Autodesk Inventor part; units mm, degrees
ref_plane "YZ Plane" through (0, 0, 0) normal (1, 0, 0) x (0, 1, 0)
ref_plane "XZ Plane" through (0, 0, 0) normal (0, 1, 0) x (-1, 0, 0)
ref_plane "XY Plane" through (0, 0, 0) normal (0, 0, 1) x (1, 0, 0)
sketch "Эскиз1" plane through (0, 0, 0) normal (0, 0, 1) x (1, 0, 0)
  line L0 (-136.1512, -7) -> (-131.1512, -2)
  line L1 (-131.1512, -2) -> (-99.224, -2)
  line L2 (-19, -2) -> (-19, -22)
  line L3 (-19, -22) -> (-24, -27)
  line L4 (-24, -27) -> (-30.8711, -27)
  line L5 (-136.1512, -27) -> (-136.1512, -7)
  line L6 (-141.1512, -58) -> (-75.0711, -58)
  line L7 (-75.0711, -58) -> (-49.0711, -32)
  line L8 (-49.0711, -32) -> (-21.9289, -32)
  line L9 (-21.9289, -32) -> (-14, -24.0711)
  line L10 (-14, -24.0711) -> (-14, 3)
  line L11 (-133.2223, 3) -> (-14, 3)
  line L12 (-133.2223, 3) -> (-141.1512, -4.9289)
  line L13 (-141.1512, -58) -> (-141.1512, -4.9289)
  line L14 (-44.9289, -42) -> (-24.8579, -42)
  line L15 (-24.8579, -42) -> (-45.8579, -63)
  line L16 (-45.8579, -63) -> (-65.9289, -63)
  line L17 (-65.9289, -63) -> (-44.9289, -42)
  line L18 (-4, 3) -> (-9, 3)
  line L19 (-9, 3) -> (-9, -26.1421)
  line L20 (-9, -26.1421) -> (-19.8579, -37)
  line L21 (-19.8579, -37) -> (-47, -37)
  line L22 (-47, -37) -> (-73, -63)
  line L23 (-73, -63) -> (-141.1512, -63)
  line L24 (-141.1512, -67.9) -> (-141.1512, -63)
  line L25 (-47.0828, -36.8) -> (-19.9407, -36.8)
  line L26 (-19.9407, -36.8) -> (-9.2, -26.0593)
  line L27 (-9.2, -26.0593) -> (-9.2, 3.2)
  line L28 (-9.2, 3.2) -> (3.2, 3.2)
  line L29 (3.2, 3.2) -> (3.2, -31.1955)
  line L30 (3.2, -31.1955) -> (-40.7045, -75.1)
  line L31 (-40.7045, -75.1) -> (-141.3512, -75.1)
  line L32 (-141.3512, -75.1) -> (-141.3512, -62.8)
  line L33 (-141.3512, -62.8) -> (-73.0828, -62.8)
  line L34 (-73.0828, -62.8) -> (-47.0828, -36.8)
  line L35 (-21.8461, -32.2) -> (-48.9882, -32.2)
  line L36 (-48.9882, -32.2) -> (-74.9882, -58.2)
  line L37 (-74.9882, -58.2) -> (-141.3512, -58.2)
  line L38 (-141.3512, -58.2) -> (-141.3512, -4.8461)
  line L39 (-141.3512, -4.8461) -> (-133.3051, 3.2)
  line L40 (-133.3051, 3.2) -> (-13.8, 3.2)
  line L41 (-13.8, 3.2) -> (-13.8, -24.1539)
  line L42 (-13.8, -24.1539) -> (-21.8461, -32.2)
  line L43 (-9, 3) -> (-14, 3)
  line L44 (-141.1512, -63) -> (-141.1512, -58)
  line L45 (-99.224, -2) -> (-93.5671, -2)
  line L46 (-93.5671, -2) -> (-86.696, -2)
  line L47 (-86.696, -2) -> (-81.0391, -2)
  line L48 (-81.0391, -2) -> (-74.168, -2)
  line L49 (-74.168, -2) -> (-68.5111, -2)
  line L50 (-68.5111, -2) -> (-61.64, -2)
  line L51 (-61.64, -2) -> (-55.9831, -2)
  line L52 (-55.9831, -2) -> (-49.112, -2)
  line L53 (-49.112, -2) -> (-43.4551, -2)
  line L54 (-43.4551, -2) -> (-36.584, -2)
  line L55 (-36.584, -2) -> (-30.9271, -2)
  line L56 (-30.9271, -2) -> (-19, -2)
  line L57 (-30.8711, -27) -> (-36.528, -27)
  line L58 (-36.528, -27) -> (-43.3991, -27)
  line L59 (-43.3991, -27) -> (-49.056, -27)
  line L60 (-49.056, -27) -> (-55.9271, -27)
  line L61 (-55.9271, -27) -> (-61.584, -27)
  line L62 (-61.584, -27) -> (-68.4551, -27)
  line L63 (-68.4551, -27) -> (-74.112, -27)
  line L64 (-74.112, -27) -> (-80.9831, -27)
  line L65 (-80.9831, -27) -> (-86.64, -27)
  line L66 (-86.64, -27) -> (-93.5111, -27)
  line L67 (-93.5111, -27) -> (-99.168, -27)
  line L68 (-99.168, -27) -> (-106.0391, -27)
  line L69 (-106.0391, -27) -> (-111.696, -27)
  line L70 (-111.696, -27) -> (-136.1512, -27)
  line L71 (-43.6868, -67.9) -> (-141.1512, -67.9)
  line L72 (-4, -28.2132) -> (-43.6868, -67.9)
  line L73 (-4, 3) -> (-4, -28.2132)
  point P0 (-9.2, 3)
  point P1 (-13.8, 3)
  point P2 (-141.1512, -58.2)
  point P3 (-141.1512, -62.8)
  dimension "d15" = 0.2
  dimension "d16" = 0.2
extrude "Выдавливание1" add sketch "Эскиз1" against normal blind 1.5 contours L37 L36 L35 L42 L41 L43 L27 L26 L25 L34 L33 L44
sketch "Эскиз2" plane through (0, 0, 0) normal (0, 0, 1) x (1, 0, 0)
  line L0 (-9.2, -26.0593) -> (-9.2, 3)
  line L1 (-9.2, 3) -> (-13.8, 3)
  line L2 (-13.8, 3) -> (-13.8, -24.1539)
  line L3 (-13.8, -24.1539) -> (-21.8461, -32.2)
  line L4 (-21.8461, -32.2) -> (-48.9882, -32.2)
  line L5 (-48.9882, -32.2) -> (-74.9882, -58.2)
  line L6 (-74.9882, -58.2) -> (-141.1512, -58.2)
  line L7 (-141.1512, -58.2) -> (-141.1512, -62.8)
  line L8 (-141.1512, -62.8) -> (-73.0828, -62.8)
  line L9 (-73.0828, -62.8) -> (-47.0828, -36.8)
  line L10 (-47.0828, -36.8) -> (-19.9407, -36.8)
  line L11 (-19.9407, -36.8) -> (-9.2, -26.0593)
  line L12 (-7.2, -26.8877) -> (-7.2, 5)
  line L13 (-7.2, 5) -> (-15.8, 5)
  line L14 (-15.8, 5) -> (-15.8, -23.3255)
  line L15 (-15.8, -23.3255) -> (-22.6745, -30.2)
  line L16 (-22.6745, -30.2) -> (-49.8167, -30.2)
  line L17 (-49.8167, -30.2) -> (-75.8167, -56.2)
  line L18 (-75.8167, -56.2) -> (-143.1512, -56.2)
  line L19 (-143.1512, -56.2) -> (-143.1512, -64.8)
  line L20 (-143.1512, -64.8) -> (-72.2544, -64.8)
  line L21 (-72.2544, -64.8) -> (-46.2544, -38.8)
  line L22 (-46.2544, -38.8) -> (-19.1123, -38.8)
  line L23 (-19.1123, -38.8) -> (-7.2, -26.8877)
  line L24 (-138.1512, -66.9) -> (-138.1512, -63)
  line L25 (-138.1512, -64.8) -> (-137.8512, -64.8)
  line L26 (-137.8512, -64.8) -> (-137.8512, -56.2)
  line L27 (-5.3, 0) -> (-14, 0)
  line L28 (-7.2, 0) -> (-7.2, -0.3)
  line L29 (-7.2, -0.3) -> (-15.8, -0.3)
  dimension "d17" = 2
  dimension "d18" = 0.3
  dimension "d19" = 0.3
extrude "Выдавливание2" add sketch "Эскиз2" along normal blind 1 contours L11 L10 L9 L8 L26 L6 L5 L4 L3 L2 L29 L0 | L0 L29 L12 L23 L22 L21 L20 L26 L8 L9 L10 L11 | L2 L3 L4 L5 L6 L26 L18 L17 L16 L15 L14 L29
mirror "Зеркальное отражение1" about plane through (-72.5256, -32.55, 1) normal (0, 0, 1) of "Выдавливание2", "Выдавливание1"
sketch "Эскиз3" plane through (0, 0, -1.5) normal (0, 0, -1) x (-1, 0, 0)
  line L0 (163, 30) -> (-28, 30)
  line L1 (-28, 30) -> (-28, -127)
  line L2 (-28, -127) -> (163, -127)
  line L3 (163, -127) -> (163, 30)
  point P0 (0, 0)
extrude "Выдавливание3" cut sketch "Эскиз3" against normal blind 2.5
sketch "Эскиз4" plane through (0, 0, 1) normal (0, 0, -1) x (-1, 0, 0)
  line L0 (39.0089, -22.15) -> (21.8668, -22.15)
  line L1 (21.8668, -22.15) -> (13.85, -14.1332)
  line L2 (13.85, -14.1332) -> (13.85, 3)
  line L3 (13.85, 3) -> (9.15, 3)
  line L4 (9.15, 3) -> (9.15, -16.08)
  line L5 (9.15, -16.08) -> (19.92, -26.85)
  line L6 (19.92, -26.85) -> (37.0621, -26.85)
  line L7 (37.0621, -26.85) -> (73.0621, -62.85)
  line L8 (73.0621, -62.85) -> (141.1512, -62.85)
  line L9 (141.1512, -62.85) -> (141.1512, -58.15)
  line L10 (141.1512, -58.15) -> (75.0089, -58.15)
  line L11 (75.0089, -58.15) -> (39.0089, -22.15)
  line L12 (9.15, -16.08) -> (9.15, -0.2)
  line L13 (6, -0.2) -> (9.15, -0.2)
  line L14 (6, -17.3848) -> (6, -0.2)
  line L15 (18.6152, -30) -> (6, -17.3848)
  line L16 (35.7574, -30) -> (18.6152, -30)
  line L17 (71.7574, -66) -> (35.7574, -30)
  line L18 (137.9512, -66) -> (71.7574, -66)
  line L19 (137.9512, -62.85) -> (137.9512, -66)
  line L20 (137.9512, -62.85) -> (73.0621, -62.85)
  line L21 (73.0621, -62.85) -> (37.0621, -26.85)
  line L22 (37.0621, -26.85) -> (19.92, -26.85)
  line L23 (19.92, -26.85) -> (9.15, -16.08)
  line L24 (13.85, -0.2) -> (13.85, -14.1332)
  line L25 (13.85, -14.1332) -> (21.8668, -22.15)
  line L26 (21.8668, -22.15) -> (39.0089, -22.15)
  line L27 (39.0089, -22.15) -> (75.0089, -58.15)
  line L28 (75.0089, -58.15) -> (137.9512, -58.15)
  line L29 (137.9512, -55) -> (137.9512, -58.15)
  line L30 (76.3137, -55) -> (137.9512, -55)
  line L31 (40.3137, -19) -> (76.3137, -55)
  line L32 (23.1716, -19) -> (40.3137, -19)
  line L33 (17, -12.8284) -> (23.1716, -19)
  line L34 (17, -0.2) -> (17, -12.8284)
  line L35 (13.85, -0.2) -> (17, -0.2)
  line L36 (137.9512, -58.15) -> (135.9512, -58.15)
  line L37 (135.9512, -58.15) -> (135.9512, -55)
  line L38 (135.9512, -55) -> (137.9512, -55)
  line L39 (137.9512, -55) -> (137.9512, -58.15)
  point P0 (0, 0)
  point P1 (135.9512, -58.15)
  dimension "d12" = 2
extrude "Выдавливание4" cut sketch "Эскиз4" against normal blind 1 contours L37 L30 L29 L10
properties part number "left_line"
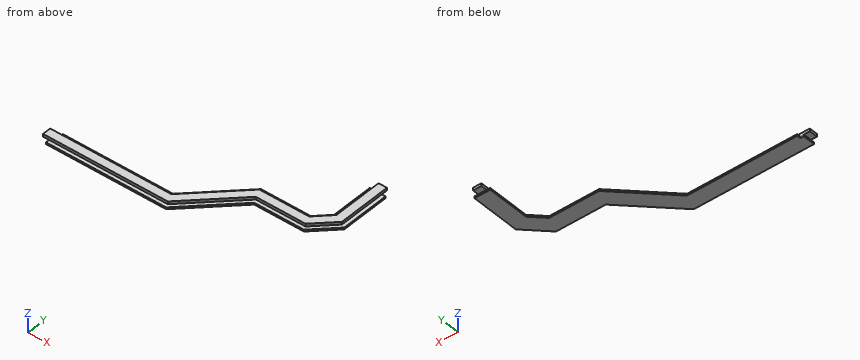
Could you check a few things on this model? Use its own coordinates, in mm. Give positions to 0.01 mm unless a question says otherwise; leave off trailing zeros. Loops run counter-clockwise (first coordinate to the right, second up) from the corner with the lowest first, then second, coordinate; pieces in that order, holes last. Notation, with made-up numbers: (-12, -37) - (-3, -37) arc R32 ccw to (-3, -1) - close; hole circle Ø7 at (88, 7.25). An arc over 180 degrees is marked (long way). Answer in a Markdown table with one row per item. Add a question column.
Q1. For pin 1 (1.2 mm diameter, centred on x = -94.5, z = 3, fed in from +Y); pin 2 (0.5 mm diameter, centred on y = -57, z = 1.5, fed in from -X); pin 3 (0.8 mm diameter, centred on x = -41, z = 1.5, fed in from +Y), each with a flat end and sliding along its axis, tell me the tip position at first contact or that it passes through.
Q2. If we section it at A-A (z = 1.5): List the corners of the cut face in (x, y) for me.
Q3. If we section it at B-B (x = -117): List the corners of the cut face in (y, z) for me, plus the area to 3 significant figures.
Q4. If we section it at C-C (y = -8): List the corners of the cut face in (x, z) for me, plus the area to 3 significant figures.
Q5. Please list where these lines run through material, in increasing order: L1, parallel to Y at x = -94, z = 2.4; L2, parallel to X at y = -23, z = 1.6; L3, parallel to X at y = -15.5, z = 2.9. Write a range as from..to.
The answers:
| question | item | result |
|---|---|---|
| 1 | pin 1 | stops at y = -58.2 |
| 1 | pin 2 | stops at x = -135.95 |
| 1 | pin 3 | stops at y = -30.2 |
| 2 | outline | (-137.85, -64.8) - (-72.25, -64.8) - (-46.25, -38.8) - (-19.11, -38.8) - (-7.2, -26.89) - (-7.2, -0.3) - (-15.8, -0.3) - (-15.8, -23.33) - (-22.67, -30.2) - (-49.82, -30.2) - (-75.82, -56.2) - (-135.95, -56.2) - (-135.95, -58.15) - (-137.85, -58.15) - close |
| 3 | outline | (-64.8, 1) - (-56.2, 1) - (-56.2, 2) - (-58.2, 2) - (-58.2, 3.5) - (-62.8, 3.5) - (-62.8, 2) - (-64.8, 2) - close |
| 3 | area | 15.5 mm^2 |
| 4 | outline | (-15.8, 1) - (-7.2, 1) - (-7.2, 2) - (-9.2, 2) - (-9.2, 3.5) - (-13.8, 3.5) - (-13.8, 2) - (-15.8, 2) - close |
| 4 | area | 15.5 mm^2 |
| 5 | L1 | y = -62.8..-58.2 |
| 5 | L2 | x = -15.8..-7.2 |
| 5 | L3 | x = -13.8..-9.2 |
